Build history of the part. All positions in model axes, mm. Face numbers are marked on the shaded views. Give positions to 0.01 mm unless a question says otherwise; leave off trailing zeros. Write each loop counter-clockwise with the first axis right and the second up, starting at its lowest first coordinate (ties: lowest second). Pieces come first, ordered by that corner, then holes. Notation, with made-up numbers: (79, -11.5) -> (89, -11.5) arc R24 cw to (89, 27.5) -> close; hole circle Ø2 at (-39.5, 26). An arc over 180 degrees is marked (long way). Put each result on its own line as item: value.
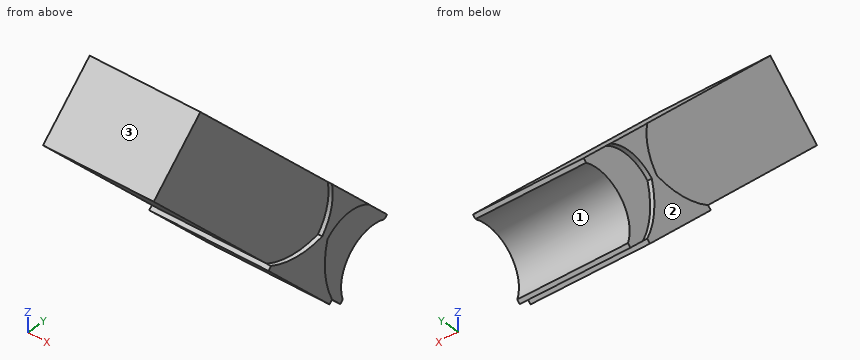
Autodesk Inventor part; units mm, degrees
ref_plane "YZ Plane" through (0, 0, 0) normal (1, 0, 0) x (0, 1, 0)
ref_plane "XZ Plane" through (0, 0, 0) normal (0, 1, 0) x (-1, 0, 0)
ref_plane "XY Plane" through (0, 0, 0) normal (0, 0, 1) x (1, 0, 0)
sketch "Sketch1" plane through (0, 0, 0) normal (1, 0, 0) x (0, 1, 0)
  line L0 (0, 0) -> (6.364, 6.364)
  line L1 (0, 0) -> (10.533, 0) construction
  line L2 (0, 0) -> (36, 0) construction
  line L3 (-19.0919, 31.8198) -> (-25.4558, 25.4558)
  line L4 (-19.0919, 31.8198) -> (6.364, 6.364)
  line L5 (-25.4558, 25.4558) -> (0, 0)
  dimension "d0" = 9
  dimension "d1" = 45
  dimension "d2" = 36
  dimension "d15" = 9
extrude "Extrusion4" add sketch "Sketch1" along normal blind 13
sketch "Sketch4" plane through (13, 0, 0) normal (1, 0, 0) x (0, 0, -1)
  line L0 (0, 0) -> (-6.364, 6.364)
  line L1 (-3.182, 3.182) -> (-1.7678, 1.7678)
  line L2 (-3.182, 3.182) -> (-1.7678, 4.5962)
  circle A0 centre (-1.7678, 4.5962) radius 4.5
  point P0 (-6.0324, 6.0324)
  point P1 (-0.3315, 0.3315)
  dimension "d18" = 2
  dimension "d19" = 2
  dimension "d20" = 9
extrude "Extrusion5" cut sketch "Sketch4" against normal blind 13 contours L0 A0 picked at (-2.8444, 1.8095)
sketch "Sketch8" plane through (13, 0, 0) normal (0, -0.7071, -0.7071) x (-1, 0, 0)
  line L0 (0, -36) -> (0, 0)
  line L1 (0, -1.9255) -> (0, -2.4255)
  line L2 (0, -2.4255) -> (-0.5, -2.4255)
  line L3 (13, -36) -> (13, 0)
  line L4 (13, -13.6899) -> (13, -14.1899)
  line L5 (13, -14.1899) -> (13.5, -14.1899)
  line L6 (13.5, -14.1899) -> (-0.5, -14.1899)
  line L7 (-0.5, -14.1899) -> (-0.5, -2.4255)
  line L8 (-0.5, -2.4255) -> (13.5, -2.4255)
  line L9 (13.5, -2.4255) -> (13.5, -14.1899)
  dimension "d31" = 0.5
  dimension "d32" = 0.5
  dimension "d33" = 0.5
  dimension "d34" = 0.5
extrude "Extrusion7" add sketch "Sketch8" along normal blind 0.5
sketch "Sketch9" plane through (13, 0, 0) normal (1, 0, 0) x (0, 0, -1)
  line L0 (-1.7151, -1.7151) -> (-10.0338, -10.0338)
  line L1 (-5.8744, -5.8744) -> (-12.2384, 0.4895)
  line L2 (-6.364, 6.364) -> (-31.8198, -19.0919)
  line L3 (-9.0564, -2.6925) -> (-8.7029, -2.3389)
  line L4 (-9.0564, -2.6925) -> (-9.41, -3.046)
  line L5 (-1.7151, -1.7151) -> (0, 0)
  arc A0 (-8.7029, -2.3389) -> (-1.7151, -1.7151) centre (-6.0417, 7.3005) ccw
  arc A1 (-10.0338, -10.0338) -> (-9.41, -3.046) centre (-19.0494, -5.7072) ccw
  arc A2 (-9.41, -3.046) -> (-14.443, -1.7151) centre (-13.3407, -7.7285) ccw
  arc A3 (-9.41, 3.3179) -> (-8.7029, -2.3389) centre (-5.3886, 0.948) ccw
  dimension "d37" = 0.5
  dimension "d38" = 0.5
  dimension "d39" = 10
  dimension "d40" = 10
extrude "Extrusion8" add sketch "Sketch9" along normal blind 0.5 and the other way blind 13.5
sketch "Sketch10" plane through (13, -25.4558, 25.4558) normal (0, -0.7071, -0.7071) x (-1, 0, 0)
  line L0 (-0.836, 22.8138) -> (15.9237, 22.8138) construction
  line L1 (15.9237, 22.8138) -> (15.9237, -0.8905) construction
  line L2 (15.9237, -0.8905) -> (-0.836, -0.8905) construction
  line L3 (-0.836, -0.8905) -> (-0.836, 22.8138) construction
  point P0 (13, 36)
decal "Decal1"
properties part number "McCrea_paza_Walle"
1) Pull direction Y, two halves, no side cores. Call the marked faces 1, 2 and 3: released by +Y, released by -Y, zero draft, split by the parting line, or undercut.
Filled sheet:
face 1: undercut
face 2: zero draft
face 3: released by -Y
2) Slice it at C-C (z = 3.5). Write the cut outline in (x, y).
Filled sheet:
outline: (-0.5, -4.21) -> (13.5, -4.21) -> (13.5, -2.37) -> (13, -2.37) -> (13, 0.44) -> (0, 0.44) -> (0, -2.37) -> (-0.5, -2.37) -> close
3) Pin check, flat tips, straight feed: pin 1 (4 mm diameter, centred on y = -7, z = 16, fed in from -X); pin 2 (3 mm diameter, centred on x = 4, y = 2, fed in from -Z); pin 3 (6 mm diameter, centred on x = 12, y = -20.5, fed in from -Z). Stop position of each tip, or through.
Filled sheet:
pin 1: x = 0
pin 2: z = 3.63
pin 3: z = 17.5
4) Slice it at A-A (x = 3). Write the cut outline in (y, z).
Filled sheet:
outline: (-25.46, 25.46) -> (-10.03, 10.03) -> (-10.39, 9.68) -> (-2.07, 1.36) -> (-1.72, 1.72) -> (0, 0) -> (0.33, 0.33) arc R4.5 cw to (6.03, 6.03) -> (6.36, 6.36) -> (-19.09, 31.82) -> close
5) Wall check: L1, parallel to X at y = -1, z = 7.5; L2, parallel to Y at x = 9.75, z = 2; L3, parallel to Z at x = 6.5, y = 4.5. Give the ranges that are in metal, low to high.
Filled sheet:
L1: 0 to 13
L2: -2.71 to 0.1
L3: 6.27 to 8.23
6) Slice it at B-B (y = -7). Write the cut outline in (x, z).
Filled sheet:
outline: (-0.5, 6.29) -> (13.5, 6.29) -> (13.5, 9.13) -> (13, 9.13) -> (13, 19.73) -> (0, 19.73) -> (0, 9.13) -> (-0.5, 9.13) -> close
7) Slice it at D-D (y = -20.5). Write the cut outline in (x, z), plus the area to 3 significant figures.
Filled sheet:
outline: (0, 20.5) -> (13, 20.5) -> (13, 30.41) -> (0, 30.41) -> close
area: 129 mm2
